Can you work these out from the model? Positions are in its coordinate system, mm. A direction names the side the tool comes from. Coordinates: 2 decimals unless noted, no trailing zeros. Write each loop counter-clockwise with the first axis right and the second up, starting at its lowest first coordinate (ties: lowest second). Pieces come first, ordered by that corner, then holes. Notation, with made-up numbers: (-1, -30.5) - (3, -30.5) arc R10 cw to (3, -17.5) - close; hole circle Ø5 at (60, -2). An arc over 180 degrees is marked (long way). Use one line per item in the form item = value. Start each with the question number.
(1) For pin 1 Ø5 at (y, z) = (10, 10) entering from +X; pin 2 Ø1 at (x, y) = (3, 24) entering from +Z; pin 3 Ø4 at (x, z) = (25, 10) entering from +Y, each with a flat end and sliding along its axis, tell me the tip position at first contact or that it passes through.
(2) On a 3-axis mill with a long thin cutter (end or side, diameter ignored), from which of +Z, -Z, +X, -X, +Y, -Y can I reach the whole of each face in a straight line? I mean faces 1 (the face through (2, 25, 10)), 2 (the face through (3, 24, 19.955)), 3 (the face through (10, 10, 17)). Say none if no direction works.
(3) If we section it at A-A on z = 10: Please give me the cut outline in (x, y), then the cut area to 3 significant figures.
(4) If I drill on probe 1 along Z at (x, y) = (8, 15.75); probe 2 along Z at (x, y) = (1.2, 10); probe 3 along Y at (x, z) = (28, 17.5), over which ranges is the centre line in solid material (lowest first)? Write a range as from..to.
(5) If we section it at D-D on y = 1.75: Please give me the cut outline in (x, z), then the cut area to 3 significant figures.
(6) If we section it at C-C on y = 10: Please give me the cut outline in (x, z), then the cut area to 3 significant figures.
(7) If we section it at B-B on x = 25: Please give me the cut outline in (y, z).
(8) Thinking about a two-plate mould opening in X: for faces 4 (the face through (25.273, 2.535, 12.082)), 5 (the face through (0, 12.3, 9.9)), 6 (the face through (14.499, 12.918, 18.521)), 7 (the face through (11, 7, 20)), which applies, pulls with the +X half, pulls with the -X half, needs draft (parallel to the pull), parting line crosses it, or undercut?
```python
from build123d import *

# Parameters (mm, degrees)
SKETCH_W        = 30
SKETCH_H        = 5
PAD_DEPTH       = 20
SKETCH001_W     = 3.989674
SKETCH001_H     = 19.955276
PAD001_DEPTH    = 20
PAD002_DEPTH    = 3
PAD003_DEPTH    = 3
SKETCH004_R     = 2.1
POCKET_DEPTH    = 10
SKETCH005_R     = 2.1
POCKET001_DEPTH = 8


with BuildPart() as part:
    # Sketch → Pad (new body)
    with BuildSketch(Plane.XY):
        with Locations((15, 2.5)):
            Rectangle(SKETCH_W, SKETCH_H)
    extrude(amount=PAD_DEPTH)

    # Sketch001 (on Face3 of Pad) → Pad001 (join)
    with BuildSketch(Plane(origin=(0, 5, 0), x_dir=(-1, 0, 0), z_dir=(0, 1, 0))):
        with Locations((-1.994837, 9.977638)):
            Rectangle(SKETCH001_W, SKETCH001_H)
    extrude(amount=PAD001_DEPTH)

    # Sketch002 (on DatumPlane) → Pad002 (join)
    with BuildSketch(Plane(origin=(0, 0, 0), x_dir=(1, 0, 0), z_dir=(0, 0, -1))):
        Polygon((0, 0), (30, 0), (0, -25), align=None)
    extrude(amount=-PAD002_DEPTH)

    # Sketch003 (on DatumPlane) → Pad003 (join)
    with BuildSketch(Plane.XY.offset(20)):
        Polygon((0, 0), (0, 25), (30, 0), align=None)
    extrude(amount=-PAD003_DEPTH)

    # Sketch004 (on Face19 of Pad003) → Pocket (cut)
    with BuildSketch(Plane.YZ.offset(3.989674)):
        with Locations((10, 10)):
            Circle(SKETCH004_R)
    extrude(amount=-POCKET_DEPTH, mode=Mode.SUBTRACT)

    # Sketch005 (on Face10 of Pocket) → Pocket001 (cut)
    with BuildSketch(Plane(origin=(0, 5, 0), x_dir=(-1, 0, 0), z_dir=(0, 1, 0))):
        with Locations((-25, 10)):
            Circle(SKETCH005_R)
    extrude(amount=-POCKET001_DEPTH, mode=Mode.SUBTRACT)


solid = part.part
```
Reported:
q1.pin_1 = 3.99
q1.pin_2 = 19.96
q1.pin_3 = through
q2.face_1 = +Z, -Z, +X, -X, +Y
q2.face_2 = +Z, +X, +Y
q2.face_3 = +X, +Y
q3.outline = (0, 0) - (22.9, 0) - (22.9, 5) - (3.99, 5) - (3.99, 7.9) - (0, 7.9) - close; (0, 12.1) - (3.99, 12.1) - (3.99, 25) - (0, 25) - close; (27.1, 0) - (30, 0) - (30, 5) - (27.1, 5) - close
q3.area = 192 mm2
q4.probe_1 = 0..3, 17..20
q4.probe_2 = 0..7.9, 12.1..20
q4.probe_3 = 0..5
q5.outline = (0, 0) - (30, 0) - (30, 20) - (0, 20) - close; hole circle Ø4.2 at (25, 10)
q5.area = 586 mm2
q6.outline = (0, 0) - (18, 0) - (18, 3) - (3.99, 3) - (3.99, 7.9) - (0, 7.9) - close; (0, 12.1) - (3.99, 12.1) - (3.99, 17) - (18, 17) - (18, 20) - (0, 20) - close
q6.area = 147 mm2
q7.outline = (0, 0) - (5, 0) - (5, 7.9) - (0, 7.9) - close; (0, 12.1) - (5, 12.1) - (5, 20) - (0, 20) - close
q8.face_4 = undercut
q8.face_5 = pulls with the -X half
q8.face_6 = pulls with the +X half
q8.face_7 = needs draft
